Model file for the job. Use its own axes, mm. A direction names the side the tool comes from. Round coordinates to 2 decimals unless told otherwise and drop trailing zeros. Order: outer loops, then holes, each group sorted by start corner. A loop starts at its lowest first (then second) coordinate and runs counter-clockwise, first axis right, second up. Notation, with made-up numbers: (89, 4) -> (96, 4) arc R16 cw to (96, 32) -> close; hole circle Ø7 at (-26, 30.25). An arc over 180 degrees is marked (long way). Answer as CSV lines item,"result".
```python
from build123d import *

# Parameters (mm, degrees)
SKETCH_1_W               = 62
SKETCH_1_H               = 90
SKETCH_1_R               = 5
SKETCH_1_R_2             = 10
EXTRUDE_1_DEPTH          = 7
SKETCH_3_R               = 10
SKETCH_3_R_2             = 5
EXTRUDE_2_DEPTH          = 7
SKETCH_4_R               = 18.5
EXTRUDE_3_DEPTH          = 20
SKETCH_5_W               = 42
SKETCH_5_H               = 18
CUT_EXTRUDE_1_DEPTH      = 7
SKETCH_7_R               = 2
EXTRUDE_5_DEPTH          = 5
SKETCH_6_R               = 4
SKETCH_6_R_2             = 2
EXTRUDE_7_DEPTH          = 12
SKETCH_18_R              = 4
CUT_EXTRUDE_8_DEPTH      = 3
CUT_EXTRUDE_3_DEPTH      = 73.124891681
CUT_EXTRUDE_3_DEPTH_BACK = 73.124891681
SKETCH_10_W              = 13.858571571
SKETCH_10_H              = 11.898979486
SKETCH_10_W_2            = 20
SKETCH_10_H_2            = 30
CUT_EXTRUDE_4_DEPTH      = 7
SKETCH_11_W              = 17.5
SKETCH_11_H              = 10
CUT_EXTRUDE_5_DEPTH      = 7
CUT_EXTRUDE_9_REACH      = 84.674
SKETCH_19_W              = 10.885621722
SKETCH_19_H              = 15
SKETCH_12_W              = 92.977348864
SKETCH_12_H              = 90
CUT_EXTRUDE_6_DEPTH      = 2
SKETCH_13_W              = 67.267412259
SKETCH_13_H              = 90
CUT_EXTRUDE_7_DEPTH      = 2
SKETCH_14_W              = 31
SKETCH_14_H              = 35
EXTRUDE_8_DEPTH          = 5
SKETCH_15_W              = 14.844505579
SKETCH_15_H              = 5
EXTRUDE_9_DEPTH          = 7
SKETCH_16_W              = 31
SKETCH_16_H              = 35
EXTRUDE_10_DEPTH         = 5
SKETCH_20_W              = 21
SKETCH_20_H              = 10
EXTRUDE_11_DEPTH         = 4
SKETCH_21_W              = 5
SKETCH_21_H              = 35
SKETCH_21_W_2            = 10
EXTRUDE_12_DEPTH         = 5
SKETCH_22_R              = 10
CUT_EXTRUDE_10_DEPTH     = 103.708324882
SKETCH_23_W              = 20
SKETCH_23_H              = 10
CUT_EXTRUDE_11_DEPTH     = 11


with BuildPart() as part:
    # Sketch 1 → Extrude 1 (new body)
    with BuildSketch(Plane(origin=(0, 0, 0), x_dir=(1, 0, 0), z_dir=(0, 1, 0))):
        Rectangle(SKETCH_1_W, SKETCH_1_H)
        with Locations(Location((-20, 20, 0), (0, 0, 270))):
            Circle(SKETCH_1_R, mode=Mode.SUBTRACT)
        with Locations(Location((20, 20, 0), (0, 0, 270))):
            Circle(SKETCH_1_R, mode=Mode.SUBTRACT)
        with Locations(Location((20, -20, 0), (0, 0, 270))):
            Circle(SKETCH_1_R, mode=Mode.SUBTRACT)
        with Locations(Location((-20, -20, 0), (0, 0, 270))):
            Circle(SKETCH_1_R, mode=Mode.SUBTRACT)
        with Locations(Location((0, 20, 0), (0, 0, 270))):
            Circle(SKETCH_1_R_2, mode=Mode.SUBTRACT)
    extrude(amount=EXTRUDE_1_DEPTH)



with BuildPart() as body_2:
    # Sketch 3 → Extrude 2 (new body)
    with BuildSketch(Plane(origin=(0, -16, 0), x_dir=(-1, 0, 0), z_dir=(0, -1, 0))):
        with BuildLine():
            Line((-31, 45), (31, 45))
            Line((31, 45), (31, -45))
            Line((31, -45), (16.155494421, -45))
            ThreePointArc((16.155494421, -45), (0, -16), (-16.155494421, -45))
            Line((-16.155494421, -45), (-31, -45))
            Line((-31, -45), (-31, 45))
        make_face()
        with Locations(Location((0, 20, 0), (0, 0, 270))):
            Circle(SKETCH_3_R, mode=Mode.SUBTRACT)
        with Locations(Location((17.5, 32.5, 0), (0, 0, 90))):
            Circle(SKETCH_3_R_2, mode=Mode.SUBTRACT)
        with Locations(Location((17.5, 7.5, 0), (0, 0, 90))):
            Circle(SKETCH_3_R_2, mode=Mode.SUBTRACT)
        with Locations(Location((-17.5, 7.5, 0), (0, 0, 90))):
            Circle(SKETCH_3_R_2, mode=Mode.SUBTRACT)
        with Locations(Location((-17.5, 32.5, 0), (0, 0, 90))):
            Circle(SKETCH_3_R_2, mode=Mode.SUBTRACT)
    extrude(amount=EXTRUDE_2_DEPTH)


with BuildPart() as part_1:
    add(part.part)

    add(body_2.part)  # Extrude 3 merges body 2
    # Sketch 4 → Extrude 3 (add)
    with BuildSketch(Plane(origin=(31, 0, 0), x_dir=(0, 0, -1), z_dir=(1, 0, 0))):
        with Locations(Location((-25, -3, 0), (0, 0, 170.667581816))):
            Circle(SKETCH_4_R)
        with Locations(Location((25, -3, 0), (0, 0, 170.667581816))):
            Circle(SKETCH_4_R)
    extrude_3 = extrude(amount=EXTRUDE_3_DEPTH)

    # Mirror 1: Extrude 3 across plane
    add(extrude_3.mirror(Plane(origin=(0, 0, 0), x_dir=(0, 0, 1), z_dir=(1, 0, 0))))

    # Sketch 5 → Cut-Extrude 1 (cut)
    with BuildSketch(Plane(origin=(0, 7, 0), x_dir=(1, 0, 0), z_dir=(0, 1, 0))):
        with Locations((0, 36)):
            Rectangle(SKETCH_5_W, SKETCH_5_H)
    extrude(amount=-CUT_EXTRUDE_1_DEPTH, mode=Mode.SUBTRACT)

    # Sketch 7 → Extrude 5 (add)
    with BuildSketch(Plane(origin=(0, 7, 0), x_dir=(1, 0, 0), z_dir=(0, 1, 0))):
        with BuildLine():
            Line((-7.141428429, 27), (-21, 27))
            Line((-21, 27), (-21, 45))
            Line((-21, 45), (-31, 45))
            Line((-31, 45), (-31, -45))
            Line((-31, -45), (31, -45))
            Line((31, -45), (31, 45))
            Line((31, 45), (21, 45))
            Line((21, 45), (21, 27))
            Line((21, 27), (7.141428429, 27))
            ThreePointArc((7.141428429, 27), (0, 10), (-7.141428429, 27))
        make_face()
        with Locations(Location((-20, 20, 0), (0, 0, 270))):
            Circle(SKETCH_7_R, mode=Mode.SUBTRACT)
        with Locations(Location((20, 20, 0), (0, 0, 270))):
            Circle(SKETCH_7_R, mode=Mode.SUBTRACT)
        with Locations(Location((20, -20, 0), (0, 0, 270))):
            Circle(SKETCH_7_R, mode=Mode.SUBTRACT)
        with Locations(Location((-20, -20, 0), (0, 0, 270))):
            Circle(SKETCH_7_R, mode=Mode.SUBTRACT)
    extrude(amount=EXTRUDE_5_DEPTH)

    # Sketch 6 → Extrude 7 (add)
    # profile 1 of 2: a face of its own
    with BuildSketch(Plane(origin=(0, 12, 0), x_dir=(1, 0, 0), z_dir=(0, 1, 0))):
        with Locations(Location((-17.5, -2.5, 0), (0, 0, 270))):
            Circle(SKETCH_6_R)
        with Locations(Location((-17.5, -2.5, 0), (0, 0, 270))):
            Circle(SKETCH_6_R_2, mode=Mode.SUBTRACT)
    # profile 2 of 2: a face of its own
    with BuildSketch(Plane(origin=(0, 12, 0), x_dir=(1, 0, 0), z_dir=(0, 1, 0))):
        with Locations(Location((17.5, -2.5, 0), (0, 0, 90))):
            Circle(SKETCH_6_R)
        with Locations(Location((17.5, -2.5, 0), (0, 0, 90))):
            Circle(SKETCH_6_R_2, mode=Mode.SUBTRACT)
    extrude(amount=EXTRUDE_7_DEPTH)

    # Sketch 18 → Cut-Extrude 8 (cut)
    with BuildSketch(Plane(origin=(0, 12, 0), x_dir=(1, 0, 0), z_dir=(0, 1, 0))):
        with Locations(Location((-20, 20, 0), (0, 0, 270))):
            Circle(SKETCH_18_R)
        with Locations(Location((20, 20, 0), (0, 0, 270))):
            Circle(SKETCH_18_R)
        with Locations(Location((20, -20, 0), (0, 0, 270))):
            Circle(SKETCH_18_R)
        with Locations(Location((-20, -20, 0), (0, 0, 270))):
            Circle(SKETCH_18_R)
    extrude(amount=-CUT_EXTRUDE_8_DEPTH, mode=Mode.SUBTRACT)

    # Sketch 9 → Cut-Extrude 3 (cut, two sides: drawn at the far end of the back side and taken through both)
    with BuildSketch(Plane(origin=(0, 0, 0), x_dir=(1, 0, 0), z_dir=(0, 1, 0)).offset(-CUT_EXTRUDE_3_DEPTH_BACK)):
        Polygon((58.168962293, 1.5), (58.168962293, 54.540507165), (0, 54.540507165), (0, 10), (17.5, 1.5), align=None)
        Polygon((0, -53.302122896), (58.168962293, -53.302122896), (58.168962293, -6.5), (17.5, -6.5), (0, -15), align=None)
    extrude(amount=CUT_EXTRUDE_3_DEPTH + CUT_EXTRUDE_3_DEPTH_BACK, mode=Mode.SUBTRACT)

    # Sketch 10 → Cut-Extrude 4 (cut)
    with BuildSketch(Plane(origin=(0, 0, 0), x_dir=(1, 0, 0), z_dir=(0, 1, 0))):
        with Locations((-14.070714215, 21.050510257)):
            Rectangle(SKETCH_10_W, SKETCH_10_H)
        with Locations((-10, -30)):
            Rectangle(SKETCH_10_W_2, SKETCH_10_H_2)
    extrude(amount=CUT_EXTRUDE_4_DEPTH, mode=Mode.SUBTRACT)

    # Sketch 11 → Cut-Extrude 5 (cut)
    with BuildSketch(Plane(origin=(0, -16, 0), x_dir=(1, 0, 0), z_dir=(0, 1, 0))):
        with Locations((-8.75, 32.5)):
            Rectangle(SKETCH_11_W, SKETCH_11_H)
        Polygon((-17.5, 12.5), (32.655458142, 12.5), (32.655458142, -18.188768946), (0, -18.188768946), (0, 2.5), (-17.5, 2.5), align=None)
    extrude(amount=-CUT_EXTRUDE_5_DEPTH, mode=Mode.SUBTRACT)

    # Sketch 19 → Cut-Extrude 9 (cut, up to next)
    with BuildSketch(Plane.XZ.offset(23), mode=Mode.PRIVATE) as cut_extrude_9_sk1:
        with Locations((-12.057189139, -20)):
            Rectangle(SKETCH_19_W, SKETCH_19_H)
    cut_extrude_9_tool1 = extrude(cut_extrude_9_sk1.sketch, amount=-CUT_EXTRUDE_9_REACH, mode=Mode.PRIVATE) & part_1.part
    add(cut_extrude_9_tool1.solids().sort_by_distance((-12.057189, -23, -20))[0], mode=Mode.SUBTRACT)

    # Sketch 12 → Cut-Extrude 6 (cut)
    with BuildSketch(Plane.XZ):
        with Locations((15.488674432, 0)):
            Rectangle(SKETCH_12_W, SKETCH_12_H)
    extrude(amount=-CUT_EXTRUDE_6_DEPTH, mode=Mode.SUBTRACT)

    # Sketch 13 → Cut-Extrude 7 (cut)
    with BuildSketch(Plane(origin=(0, -16, 0), x_dir=(1, 0, 0), z_dir=(0, 1, 0))):
        with Locations((2.63370613, 0)):
            Rectangle(SKETCH_13_W, SKETCH_13_H)
    extrude(amount=-CUT_EXTRUDE_7_DEPTH, mode=Mode.SUBTRACT)

    # Sketch 14 → Extrude 8 (add)
    with BuildSketch(Plane(origin=(0, 0, -45), x_dir=(-1, 0, 0), z_dir=(0, 0, -1))):
        with Locations((15.5, -5.5)):
            Rectangle(SKETCH_14_W, SKETCH_14_H)
    extrude(amount=EXTRUDE_8_DEPTH)

    # Sketch 15 → Extrude 9 (add)
    with BuildSketch(Plane.XY.offset(45)):
        Polygon((0, 12), (0, 7), (-20, 7), (-20, 2), (-31, 2), (-31, 12), align=None)
        with Locations((-23.577747211, -20.5)):
            Rectangle(SKETCH_15_W, SKETCH_15_H)
    extrude(amount=EXTRUDE_9_DEPTH)

    # Sketch 16 → Extrude 10 (add)
    with BuildSketch(Plane.XY.offset(52)):
        with Locations((-15.5, -5.5)):
            Rectangle(SKETCH_16_W, SKETCH_16_H)
    extrude(amount=EXTRUDE_10_DEPTH)

    # Sketch 20 → Extrude 11 (add)
    with BuildSketch(Plane.XZ.offset(-2)):
        with Locations((-10.5, -40)):
            Rectangle(SKETCH_20_W, SKETCH_20_H)
    extrude(amount=-EXTRUDE_11_DEPTH)

    # Sketch 21 → Extrude 12 (add)
    with BuildSketch(Plane.ZY.offset(31)):
        with Locations((0, -5.5)):
            Rectangle(SKETCH_21_W, SKETCH_21_H)
        with Locations((52, -5.5)):
            Rectangle(SKETCH_21_W_2, SKETCH_21_H)
    extrude(amount=EXTRUDE_12_DEPTH)

    # Sketch 22 → Cut-Extrude 10 (cut, through all)
    with BuildSketch(Plane.ZY.offset(51)):
        with Locations((-25, -3)):
            Circle(SKETCH_22_R)
        with Locations((25, -3)):
            Circle(SKETCH_22_R)
    extrude(amount=-CUT_EXTRUDE_10_DEPTH, mode=Mode.SUBTRACT)

    # Sketch 23 → Cut-Extrude 11 (cut)
    with BuildSketch(Plane(origin=(-20, 0, 0), x_dir=(0, 0, -1), z_dir=(1, 0, 0))):
        with Locations((-25, 2)):
            Rectangle(SKETCH_23_W, SKETCH_23_H)
        Polygon((15, -3), (35, -3), (35, 7), (15.101020514, 7), align=None)
    extrude(amount=-CUT_EXTRUDE_11_DEPTH, mode=Mode.SUBTRACT)


solid = part_1.part
```
Q1. Flat gauge pins, fed straight in: pin 1 (2.5 mm diameter, centred on y = -5.5, z = 49, fed in from +X); pin 2 (6.5 mm diameter, centred on x = -20, z = -20, fed in from +Y); pin 3 (4 mm diameter, centred on x = 14.5, y = 10, fed in from +Z); pin 4 (4 mm diameter, centred on y = 1.5, z = 20.5, fed in from +X). Where does each tip first touch, or does it go through?
Checks:
pin 1,"x = -31"
pin 2,"y = 9"
pin 3,"z = 8.93"
pin 4,"through"
Q2. Wall check: L1, parallel to Z at x = -20, y = 7.95; L2, parallel to Z at x = -45, y = -3; L3, parallel to Z at x = -41, y = 12. Give the ranges that are in metal, low to high. Write a range as [from, to].
Checks:
L1,"[-50, -45], [-27, -22], [-18, 18], [22, 57]"
L2,"[-43.5, -35], [-15, -6.5], [6.5, 15], [35, 43.5]"
L3,"[-35.83, -14.17], [14.17, 35.83]"
Q3. Saw through at D-D (y = -3). State how many separate pieces and enclosed holes the cut face has, plus the area to 4 significant figures.
Checks:
separate pieces,"7"
enclosed holes,"0"
area,"1,065 mm²"
Q4. Saw through at C-C (z = 20). Write the cut outline in (x, y).
Checks:
outline,"(-51, -20.81) -> (-31, -20.81) -> (-31, -23) -> (-11.66, -23) -> (-11.66, -18) -> (-31, -18) -> (-31, -11.66) -> (-51, -11.66) -> close; (-51, 5.66) -> (-31, 5.66) -> (-31, 7) -> (-22, 7) -> (-22, 9) -> (-24, 9) -> (-24, 12) -> (-31, 12) -> (-31, 14.81) -> (-51, 14.81) -> close; (-18, 7) -> (0, 7) -> (0, 12) -> (-16, 12) -> (-16, 9) -> (-18, 9) -> close"
Q5. Mould opens along X. For faces 6 (the flat face through (-15, -5, -50)), 7 (the flat face through (-21, 9, -36)), 8 (the flat face through (-51, 6, 32)), 9 (the flat face through (-21, 9, -22)) say: +X half, -X half, draft (parallel to the pull), parting line (faces both ways), or undercut.
Checks:
face 6,"draft"
face 7,"+X half"
face 8,"-X half"
face 9,"undercut"
Q6. Tool access for faces 1 (the flat face through (-31, -8, 0)), 2 (the cylindrical face through (-22.5, -20.5, -7.4)), 3 (the cylindrical face through (-14.127, 17.916, 4.65)), 4 (the flat face through (0, -6, -46)), 5 (the flat face through (-31, 8, 44)): list every direction of +Z, -Z, +X, -X, +Y, -Y with a clear straight run to the whole face (end or side of a thin tool).
Checks:
face 1,"+X"
face 2,"+X, -Y"
face 3,"+Y"
face 4,"-Z, +X, +Y, -Y"
face 5,"-X, +Y"
Q7. Saw through at B-B (y = 21). Write the cut outline in (x, z), plus the area to 3 significant figures.
Checks:
outline,"circle Ø8 at (-17.5, 2.5); circle Ø8 at (17.5, 2.5); hole circle Ø4 at (-17.5, 2.5); hole circle Ø4 at (17.5, 2.5)"
area,"75.4 mm²"
Q8. Saw through at A-A (y = 14). Write the cut outline in (x, z), plus the area to 3 significant figures.
Checks:
outline,"(-51, -32.3) -> (-31, -32.3) -> (-31, -17.7) -> (-51, -17.7) -> close; (-51, 17.7) -> (-31, 17.7) -> (-31, 32.3) -> (-51, 32.3) -> close; circle Ø8 at (-17.5, 2.5); circle Ø8 at (17.5, 2.5); hole circle Ø4 at (-17.5, 2.5); hole circle Ø4 at (17.5, 2.5)"
area,"659 mm²"
